The model under review builds one solid part; all positions refer to its coordinate system, in mm. Round coordinates to 2 decimals unless told otherwise and drop trailing zeros. Loops run counter-clockwise (first coordinate to the right, second up) from the corner with the lowest first, then second, coordinate; pieces in that order, holes last. Notation, with made-up numbers: (10, 8.25) - (34, 8.25) arc R16 cw to (34, 27.25) - close; hole circle Ø4 at (47, -15.5). An arc over 180 degrees is marked (long way). Answer as CSV lines item,"result".
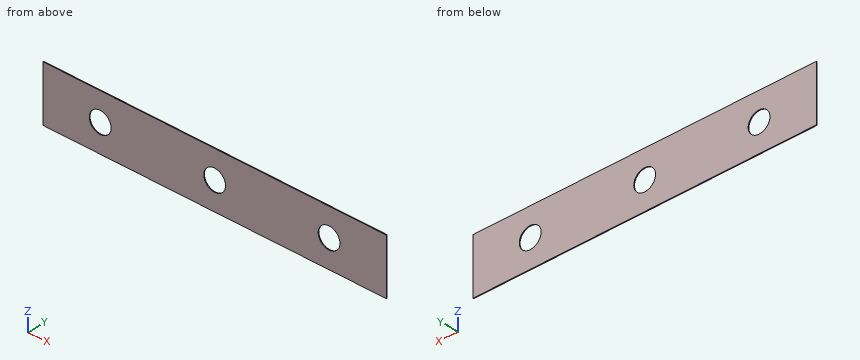
from build123d import *

# Parameters (mm, degrees)
SKETCH1_W           = 76.2
SKETCH1_H           = 12.7
BOSS_EXTRUDE1_DEPTH = 0.1778
SKETCH2_R           = 2.41935
CUT_EXTRUDE1_DEPTH  = 1.1778


with BuildPart() as part:
    # Sketch1 → Boss-Extrude1 (new body)
    with BuildSketch(Plane(origin=(0, 0, 0), x_dir=(1, 0, 0), z_dir=(0, 1, 0))):
        Rectangle(SKETCH1_W, SKETCH1_H)
    extrude(amount=BOSS_EXTRUDE1_DEPTH)

    # Sketch2 → Cut-Extrude1 (cut, through all)
    with BuildSketch(Plane(origin=(0, 0.1778, 0), x_dir=(1, 0, 0), z_dir=(0, 1, 0))):
        Circle(SKETCH2_R)
        with Locations((-25.4, 0)):
            Circle(SKETCH2_R)
        with Locations((25.4, 0)):
            Circle(SKETCH2_R)
    extrude(amount=-CUT_EXTRUDE1_DEPTH, mode=Mode.SUBTRACT)


solid = part.part
1. Take a section at C-C (x = 25.4). State the section outline as (y, z) points.
Numbers:
outline,"(0, -6.35) - (0.18, -6.35) - (0.18, -2.42) - (0, -2.42) - close; (0, 2.42) - (0.18, 2.42) - (0.18, 6.35) - (0, 6.35) - close"
2. Take a section at B-B (z = 0). State the section outline as (x, y) points, plus the area to 3 significant figures.
Numbers:
outline,"(-38.1, 0) - (-27.82, 0) - (-27.82, 0.18) - (-38.1, 0.18) - close; (-22.98, 0) - (-2.42, 0) - (-2.42, 0.18) - (-22.98, 0.18) - close; (2.42, 0) - (22.98, 0) - (22.98, 0.18) - (2.42, 0.18) - close; (27.82, 0) - (38.1, 0) - (38.1, 0.18) - (27.82, 0.18) - close"
area,"11.0 mm²"
3. Take a section at A-A (y = 0.1). State the section outline as (x, z) points, plus the area to 3 significant figures.
Numbers:
outline,"(-38.1, -6.35) - (38.1, -6.35) - (38.1, 6.35) - (-38.1, 6.35) - close; hole circle Ø4.84 at (-25.4, 0); hole circle Ø4.84 at (0, 0); hole circle Ø4.84 at (25.4, 0)"
area,"913 mm²"
4. Wall thickness on probe 1 along X at (y, z) = (0.1, 0); probe 2 along Z at (x, y) = (0, 0.1); probe 3 along X at (y, z) = (0.1, 1.75): over which ranges is each line inside the solid? List them lowest first.
Numbers:
probe 1,"x = -38.1 to -27.82, -22.98 to -2.42, 2.42 to 22.98, 27.82 to 38.1"
probe 2,"z = -6.35 to -2.42, 2.42 to 6.35"
probe 3,"x = -38.1 to -27.07, -23.73 to -1.67, 1.67 to 23.73, 27.07 to 38.1"
5. Take a section at D-D (x = 1.5). State the section outline as (y, z) points.
Numbers:
outline,"(0, -6.35) - (0.18, -6.35) - (0.18, -1.9) - (0, -1.9) - close; (0, 1.9) - (0.18, 1.9) - (0.18, 6.35) - (0, 6.35) - close"
6. Clearance check with a flat-ended pin moving along its axis: pin 1 (4.5 mm diameter, centred on x = 25.4, z = 0, fed in from +Y). State where the tip first meets the part, or that it passes through.
Numbers:
pin 1,"passes through"
